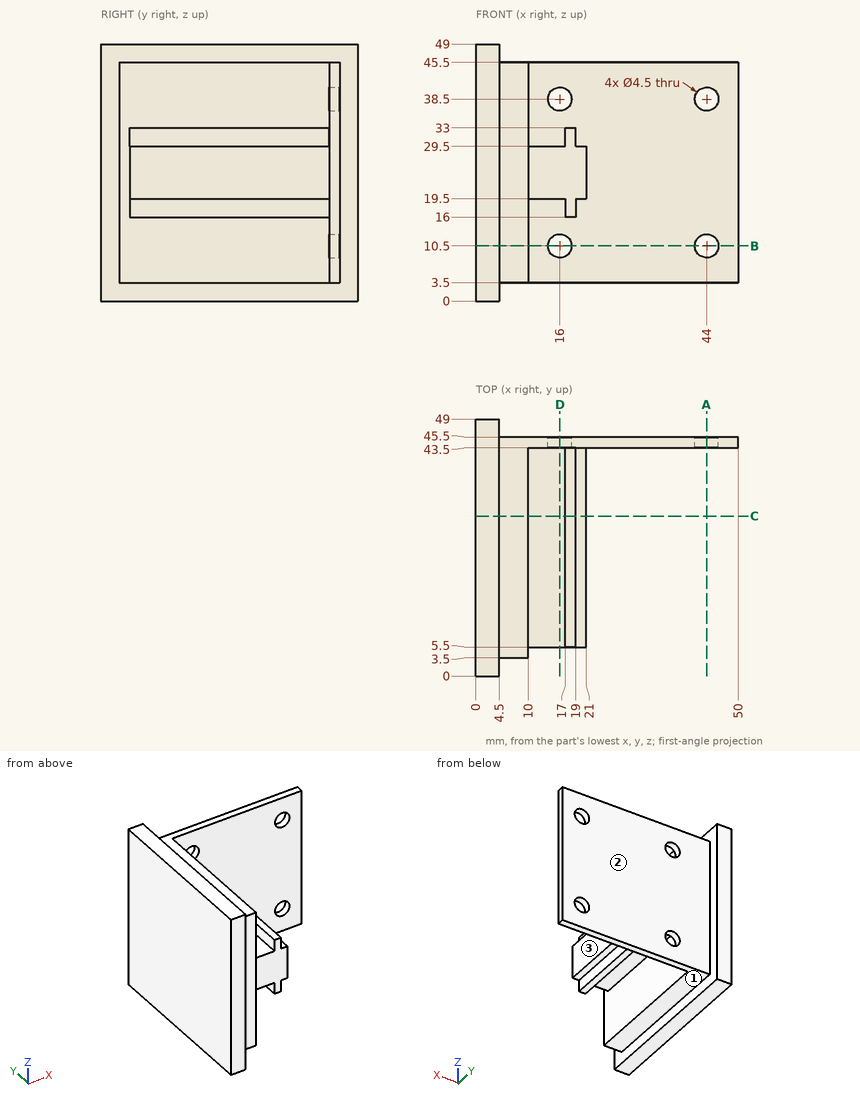
Drawing for the job (mm, zero at the part's lowest x, y, z). A direction names the side the tool comes from. Give positions to 0.01 mm unless a question says otherwise; leave off trailing zeros. Order: outer loops, then holes, each group sorted by start corner. A loop starts at its lowest first (then second) coordinate and runs counter-clockwise, first axis right, second up. Notation, with made-up numbers: M 34.25,-5 L 81.25,-5 A20 cw 81.25,16 Z; hole C -8.5,54.5 d5. An arc over 180 degrees is marked long. Put each result on its own line as item: value. Start each with the question number.
(1) Flat gauge pins, fed straight in: pin 1 Ø1 at (x, z) = (42.5, 5) entering from +Y; pin 2 Ø4 at (x, z) = (19.5, 23.5) entering from -Y; pin 3 Ø1.6 at (x, y) = (18, 28) entering from -Z. Where does each tip first touch, or does it go through?
(2) Saw through at B-B, the plane z = 10.5. Write the cut outline in (x, y), then the cut area to 4 significant figures.
(3) Saw through at A-A, the plane x = 44. Write the cut outline in (y, z), then the cut area to 3 significant figures.
(4) Drill centre lines: line 1 along Z through (x, y) = (44, 44.55); line 2 along X through (y, z) = (45.1, 38.5); line 3 along X through (y, z) = (18.5, 19). Where is each one in solid material? Low to high.
(5) Saw through at D-D, the plane x = 16. Write the cut outline in (y, z), then the cut area to 3 significant figures.
(6) Saw through at C-C, the plane y = 30.5. Write the cut outline in (x, z).
(7) Which spindle directions (+Z, -Z, +X, -X, +Y, -Y) get a long thin tool onto all of the face, cutting with end or side? Do the marked faces 1, 2 and 3. Say none if no direction does.
Check result:
1. pin 1: stops at y = 45.5
1. pin 2: stops at y = 5.5
1. pin 3: stops at z = 16
2. outline: M 0,0 L 4.5,0 L 4.5,3.5 L 10,3.5 L 10,43.5 L 13.75,43.5 L 13.75,45.5 L 4.5,45.5 L 4.5,49 L 0,49 Z; M 18.25,43.5 L 41.75,43.5 L 41.75,45.5 L 18.25,45.5 Z; M 46.25,43.5 L 50,43.5 L 50,45.5 L 46.25,45.5 Z
2. area: 513.5 mm2
3. outline: M 43.5,3.5 L 45.5,3.5 L 45.5,8.25 L 43.5,8.25 Z; M 43.5,12.75 L 45.5,12.75 L 45.5,36.25 L 43.5,36.25 Z; M 43.5,40.75 L 45.5,40.75 L 45.5,45.5 L 43.5,45.5 Z
3. area: 66.0 mm2
4. line 1: z = 3.5 to 8.25, 12.75 to 36.25, 40.75 to 45.5
4. line 2: x = 0 to 13.75, 18.25 to 41.75, 46.25 to 50
4. line 3: x = 0 to 10, 17 to 19
5. outline: M 5.5,19.5 L 43.5,19.5 L 43.5,12.75 L 45.5,12.75 L 45.5,36.25 L 43.5,36.25 L 43.5,29.5 L 5.5,29.5 Z; M 43.5,3.5 L 45.5,3.5 L 45.5,8.25 L 43.5,8.25 Z; M 43.5,40.75 L 45.5,40.75 L 45.5,45.5 L 43.5,45.5 Z
5. area: 446 mm2
6. outline: M 0,0 L 4.5,0 L 4.5,3.5 L 10,3.5 L 10,19.5 L 17,19.5 L 17,16 L 19,16 L 19,19.5 L 21,19.5 L 21,29.5 L 19,29.5 L 19,33 L 17,33 L 17,29.5 L 10,29.5 L 10,45.5 L 4.5,45.5 L 4.5,49 L 0,49 Z
7. face 1: -Z, +X, +Y, -Y
7. face 2: +Z, -Z, +X, +Y
7. face 3: +Z, -Z, +X, -Y
